Part model, mm, in its own coordinate system. A direction names the side the tool comes from. Coordinates: 2 decimals unless noted, no trailing zeros. Write each loop counter-clockwise with the first axis right and the second up, starting at its lowest first coordinate (ties: lowest second). Pieces come first, ordered by that corner, then holes. Notation, with made-up numbers: (-16.5, 13) -> (41.5, 13) arc R16 ccw to (41.5, 41) -> close; hole circle Ø9 at (56, 5). An arc over 180 degrees is marked (long way). Write item = value, one per line.
from build123d import *

# Parameters (mm, degrees)
EXTRUDE_1_DEPTH        = 5
HOLE_WIZARD_M5_1_D     = 4.2
HOLE_WIZARD_M5_1_DEPTH = 5
SKETCH_4_R             = 1.6
CUT_EXTRUDE_1_DEPTH    = 10
SKETCH_5_R             = 1.6
CUT_EXTRUDE_2_DEPTH    = 10
SKETCH_6_R             = 6
CUT_EXTRUDE_3_DEPTH    = 10
CHAMFER_1_SIZE         = 2
CUT_EXTRUDE_4_DEPTH    = 6
CHAMFER_2_SIZE         = 3
SKETCH_8_R             = 1.3
CUT_EXTRUDE_5_DEPTH    = 6
SKETCH_9_R             = 1.3
CUT_EXTRUDE_6_DEPTH    = 6
CUT_EXTRUDE_8_DEPTH    = 10
FILLET_1_R             = 3
SKETCH_12_W            = 15
SKETCH_12_H            = 14
CUT_EXTRUDE_9_DEPTH    = 10
FILLET_2_R             = 2
SKETCH_13_W            = 8
SKETCH_13_H            = 6.5
CUT_EXTRUDE_10_DEPTH   = 10
FILLET_3_R             = 1
SKETCH_14_R            = 1.3
CUT_EXTRUDE_11_DEPTH   = 10
SKETCH_15_W            = 10
SKETCH_15_H            = 5
CUT_EXTRUDE_12_DEPTH   = 10
FILLET_4_R             = 1


with BuildPart() as part:
    # 草图1 → 凸台-拉伸1 (new body)
    with BuildSketch(Plane(origin=(0, 0, 0), x_dir=(1, 0, 0), z_dir=(0, 1, 0))):
        with BuildLine():
            Line((-28.5, 0), (28.5, 0))
            Line((28.5, 0), (28.5, -51))
            ThreePointArc((28.5, -51), (0, -79.5), (-28.5, -51))
            Line((-28.5, -51), (-28.5, 0))
        make_face()
    extrude(amount=EXTRUDE_1_DEPTH)

    # M5 螺纹孔1
    with Locations(Plane(origin=(19, 5, 8), x_dir=(0, 0, 1), z_dir=(0, 1, 0))):
        with Locations((0, 0), (0, -38)):
            Hole(HOLE_WIZARD_M5_1_D / 2, depth=HOLE_WIZARD_M5_1_DEPTH)

    # 草图4 → 切除-拉伸1 (cut)
    with BuildSketch(Plane.XZ):
        with Locations((-13.435028843, 64.435028843)):
            Circle(SKETCH_4_R)
        with Locations((13.435028843, 64.435028843)):
            Circle(SKETCH_4_R)
        with Locations((13.435028843, 37.564971157)):
            Circle(SKETCH_4_R)
        with Locations((-13.435028843, 37.564971157)):
            Circle(SKETCH_4_R)
    extrude(amount=-CUT_EXTRUDE_1_DEPTH, mode=Mode.SUBTRACT)

    # 草图5 → 切除-拉伸2 (cut)
    with BuildSketch(Plane.XZ):
        with Locations((0, 64.5)):
            Circle(SKETCH_5_R)
        with Locations((11.691342951, 57.75)):
            Circle(SKETCH_5_R)
        with Locations((11.691342951, 44.25)):
            Circle(SKETCH_5_R)
        with Locations((0, 37.5)):
            Circle(SKETCH_5_R)
        with Locations((-11.691342951, 44.25)):
            Circle(SKETCH_5_R)
        with Locations((-11.691342951, 57.75)):
            Circle(SKETCH_5_R)
    extrude(amount=-CUT_EXTRUDE_2_DEPTH, mode=Mode.SUBTRACT)

    # 草图6 → 切除-拉伸3 (cut)
    with BuildSketch(Plane.XZ):
        with Locations((0, 51)):
            Circle(SKETCH_6_R)
    extrude(amount=-CUT_EXTRUDE_3_DEPTH, mode=Mode.SUBTRACT)

    # 倒角1
    chamfer_1_edges = [part.edges().sort_by_distance(p)[0] for p in [
        (-28.5, 2.5, 0),
        (28.5, 2.5, 0),
    ]]
    chamfer(chamfer_1_edges, length=CHAMFER_1_SIZE)

    # 草图7 → 切除-拉伸4 (cut, through all)
    with BuildSketch(Plane(origin=(0, 5, 0), x_dir=(1, 0, 0), z_dir=(0, 1, 0))):
        Polygon((-24, 0), (-24, -12), (-28.5, -42), (-28.5, -2), (-26.5, 0), align=None)
        Polygon((28.5, -2), (28.5, -42), (24, -12), (24, 0), (26.5, 0), align=None)
    extrude(amount=-CUT_EXTRUDE_4_DEPTH, mode=Mode.SUBTRACT)

    # 倒角2
    chamfer_2_edges = [part.edges().sort_by_distance(p)[0] for p in [
        (-24, 2.5, 0),
        (24, 2.5, 0),
    ]]
    chamfer(chamfer_2_edges, length=CHAMFER_2_SIZE)

    # 草图8 → 切除-拉伸5 (cut, through all)
    with BuildSketch(Plane(origin=(0, 5, 0), x_dir=(1, 0, 0), z_dir=(0, 1, 0))):
        with Locations((-21.650635095, -63.5)):
            Circle(SKETCH_8_R)
        with Locations((21.650635095, -63.5)):
            Circle(SKETCH_8_R)
    extrude(amount=-CUT_EXTRUDE_5_DEPTH, mode=Mode.SUBTRACT)

    # 草图9 → 切除-拉伸6 (cut, through all)
    with BuildSketch(Plane(origin=(0, 5, 0), x_dir=(1, 0, 0), z_dir=(0, 1, 0))):
        with Locations((-21, -18)):
            Circle(SKETCH_9_R)
        with Locations((21, -18)):
            Circle(SKETCH_9_R)
    extrude(amount=-CUT_EXTRUDE_6_DEPTH, mode=Mode.SUBTRACT)

    # 草图11 → 切除-拉伸8 (cut)
    with BuildSketch(Plane(origin=(0, 5, 0), x_dir=(1, 0, 0), z_dir=(0, 1, 0))):
        Polygon((-7.5, 0), (0, -6), (7.5, 0), align=None)
    extrude(amount=-CUT_EXTRUDE_8_DEPTH, mode=Mode.SUBTRACT)

    # 圆角1
    fillet_1_edges = [part.edges().sort_by_distance(p)[0] for p in [
        (-7.5, 2.5, 0),
        (7.5, 2.5, 0),
        (0, 2.5, 6),
    ]]
    fillet(fillet_1_edges, radius=FILLET_1_R)

    # 草图12 → 切除-拉伸9 (cut)
    with BuildSketch(Plane(origin=(0, 5, 0), x_dir=(1, 0, 0), z_dir=(0, 1, 0))):
        with Locations((0, -66)):
            Rectangle(SKETCH_12_W, SKETCH_12_H)
    extrude(amount=-CUT_EXTRUDE_9_DEPTH, mode=Mode.SUBTRACT)

    # 圆角2
    fillet_2_edges = [part.edges().sort_by_distance(p)[0] for p in [
        (-7.5, 2.5, 73),
        (-7.5, 2.5, 59),
        (7.5, 2.5, 59),
        (7.5, 2.5, 73),
    ]]
    fillet(fillet_2_edges, radius=FILLET_2_R)

    # 草图13 → 切除-拉伸10 (cut)
    with BuildSketch(Plane.XZ):
        with Locations((0, 76.25)):
            Rectangle(SKETCH_13_W, SKETCH_13_H)
    extrude(amount=-CUT_EXTRUDE_10_DEPTH, mode=Mode.SUBTRACT)

    # 圆角3
    fillet_3_edges = [part.edges().sort_by_distance(p)[0] for p in [
        (4, 2.5, 73),
        (-4, 2.5, 73),
        (-4, 2.5, 79.217902119),
        (4, 2.5, 79.217902119),
    ]]
    fillet(fillet_3_edges, radius=FILLET_3_R)

    # 草图14 → 切除-拉伸11 (cut)
    with BuildSketch(Plane.XZ):
        with Locations((-9, 75)):
            Circle(SKETCH_14_R)
        with Locations((9, 75)):
            Circle(SKETCH_14_R)
    extrude(amount=-CUT_EXTRUDE_11_DEPTH, mode=Mode.SUBTRACT)

    # 草图15 → 切除-拉伸12 (cut)
    with BuildSketch(Plane(origin=(0, 5, 0), x_dir=(1, 0, 0), z_dir=(0, 1, 0))):
        with Locations((0, -19.5)):
            Rectangle(SKETCH_15_W, SKETCH_15_H)
    extrude(amount=-CUT_EXTRUDE_12_DEPTH, mode=Mode.SUBTRACT)

    # 圆角4
    fillet_4_edges = [part.edges().sort_by_distance(p)[0] for p in [
        (-5, 2.5, 22),
        (-5, 2.5, 17),
        (5, 2.5, 17),
        (5, 2.5, 22),
    ]]
    fillet(fillet_4_edges, radius=FILLET_4_R)


solid = part.part
Q1. Pin check, flat tips, straight feed: pin 1 (1.5 mm diameter, centred on x = 1, y = 1.5, fed in from -Z); pin 2 (1.5 mm diameter, centred on y = 3.5, z = 19, fed in from +X); pin 3 (1.5 mm diameter, centred on y = 1.5, z = 39, fed in from -X); pin 4 (2 mm diameter, centred on x = 21.65, z = 63.5, fed in from +Y). Stop position of each tip, or through.
Model answer:
pin_1 = 4.59
pin_2 = 25.16
pin_3 = -28.16
pin_4 = through
Q2. Saw through at C-C on y = 0.8. Count the separate pieces of the cut face and the enclosed holes in it, and give its area (3 significant figures).
Model answer:
separate_pieces = 1
enclosed_holes = 19
area = 3,330 mm²
Q3. Mould opens along X. For faces 3 (the face through (-10.83, 2.46, 59.1)), 4 (the face through (-23, 3, 2)), 5 (the face through (0, 0, 30)) say: released by +X, released by -X, zero draft, split by the parting line, or undercut.
Model answer:
face_3 = undercut
face_4 = released by -X
face_5 = zero draft
Q4. Which spindle directions (+Z, -Z, +X, -X, +Y, -Y) get a long thin tool onto all of the face, cutting with end or side? Do faces 1 (the face through (6.93, 2.46, 72.4)), 2 (the face through (26.28, 2.54, 27.21)). Say none if no direction does.
Model answer:
face_1 = +Y, -Y
face_2 = -Z, +X, +Y, -Y
Q5. Saw through at D-D on z = 11. Give the cut face in (x, y).
Model answer:
outline = (-24, 0) -> (24, 0) -> (24, 5) -> (-24, 5) -> close
Q6. Saw through at A-A on x = 0. Give the cut face in (y, z).
Model answer:
outline = (0, 5.16) -> (5, 5.16) -> (5, 17) -> (0, 17) -> close; (0, 22) -> (5, 22) -> (5, 35.9) -> (0, 35.9) -> close; (0, 39.1) -> (5, 39.1) -> (5, 45) -> (0, 45) -> close; (0, 57) -> (5, 57) -> (5, 59) -> (0, 59) -> close
Q7. Saw through at B-B on z = 72. Give the cut face in (x, y), and give its area (3 significant figures).
Model answer:
outline = (-19.27, 0) -> (-7.23, 0) -> (-7.23, 5) -> (-19.27, 5) -> close; (7.23, 0) -> (19.27, 0) -> (19.27, 5) -> (7.23, 5) -> close
area = 120 mm²
Q8. Probe line 1 (Z direction, x = 0, y = 1.75); line 2 (Z direction, x = -13, y = 0.85); line 3 (Z direction, x = 12, y = 3.35). List the from-to ranges inside material, lowest first. Write a range as from..to.
Model answer:
line_1 = 5.16..17, 22..35.9, 39.1..45, 57..59
line_2 = 0..36.03, 39.1..43.33, 45.17..56.83, 58.67..62.9, 65.97..76.36
line_3 = 0..36.86, 38.27..42.68, 45.82..56.18, 59.32..63.73, 65.14..76.85
